```python
from build123d import *

# Parameters (mm, degrees)
F0_W     = 381
F0_H     = 127
F0_H_2   = 5.08
F1_DEPTH = 666.75


with BuildPart() as f1:
    # F0 (on Front) → F1 (new body)
    with BuildSketch(Plane.XZ):
        Polygon((-518.244692, 429.259082), (-518.244692, 434.339082), (-562.694692, 434.339082), (-562.694692, -448.310918), (-518.244692, -448.310918), (-518.244692, -321.310918), align=None)
        with Locations((-327.744692, -384.810918)):
            Rectangle(F0_W, F0_H)
        Polygon((-92.794692, 434.339082), (-137.244692, 434.339082), (-137.244692, 429.259082), (-137.244692, -321.310918), (-137.244692, -448.310918), (-92.794692, -448.310918), align=None)
        with Locations((-327.744692, 431.799082)):
            Rectangle(F0_W, F0_H_2)
    extrude(amount=-F1_DEPTH)


solid = f1.part
```
Part model, mm, in its own coordinate system. A direction names the side the tool comes from. Round coordinates to 2 decimals unless told otherwise and drop trailing zeros. Loops run counter-clockwise (first coordinate to the right, second up) from the corner with the lowest first, then second, coordinate; pieces in that order, holes last. Notation, with made-up numbers: (29.25, 5) -> (81.25, 5) arc R18 ccw to (81.25, 25) -> close; hole circle Ø11 at (33.5, -7.75). An arc over 180 degrees is marked (long way). Use one line per item in the form item = value. Start each with the question number.
Item 1: Tool access for faces 4 (the flat face through (-324, 329, 434.339)), 5 (the flat face through (-518.245, 329, 49)): list every direction of +Z, -Z, +X, -X, +Y, -Y with a clear straight run to the whole face (end or side of a thin tool).
Item 2: Two-plate mould, pull along X, no slides. Class faces 1 (the flat face through (-520, 0, -168)), 2 (the flat face through (-330, 329, -321.311)), 3 (the flat face through (-92.795, 329, -13)): released by +X, released by -X, zero draft, split by the parting line, or undercut.
Item 3: Band-saw the part on C-C (x = -420). List the corners of the cut face in (y, z).
Item 4: Drill centre lines: line 1 along X through (y, z) = (305.5, 309); line 2 along Z through (x, y) = (-299.5, 505.5). Where is each one in solid material? Low to high.
Item 5: Band-saw the part on A-A (z = 147). List the corners of the cut face in (x, y), plus the area to 3 significant figures.
Item 6: Band-saw the part on B-B (y = 78). List the corners of the cut face in (x, z), plus the area to 3 significant figures.
Data:
q1.face_4 = +Z, +X, -X, +Y, -Y
q1.face_5 = +Y, -Y
q2.face_1 = zero draft
q2.face_2 = undercut
q2.face_3 = released by +X
q3.outline = (0, -448.31) -> (666.75, -448.31) -> (666.75, -321.31) -> (0, -321.31) -> close; (0, 429.26) -> (666.75, 429.26) -> (666.75, 434.34) -> (0, 434.34) -> close
q4.line_1 = -562.69 to -518.24, -137.24 to -92.79
q4.line_2 = -448.31 to -321.31, 429.26 to 434.34
q5.outline = (-562.69, 0) -> (-518.24, 0) -> (-518.24, 666.75) -> (-562.69, 666.75) -> close; (-137.24, 0) -> (-92.79, 0) -> (-92.79, 666.75) -> (-137.24, 666.75) -> close
q5.area = 59,300 mm^2
q6.outline = (-562.69, -448.31) -> (-92.79, -448.31) -> (-92.79, 434.34) -> (-562.69, 434.34) -> close; hole (-518.24, -321.31) -> (-137.24, -321.31) -> (-137.24, 429.26) -> (-518.24, 429.26) -> close
q6.area = 129,000 mm^2
